Work out the finished part from the listing and answer in its coordinate system (mm). A direction names the side the tool comes from. Round coordinates to 2 decimals unless told otherwise and drop trailing zeros. Order: outer loops, then holes, each group sorted by start corner. A loop starts at its lowest first (then second) coordinate and runs counter-clockwise, first axis right, second up.
from build123d import *

# Parameters (mm, degrees)
F0_W     = 30
F0_H     = 30
F1_DEPTH = 2
F2_SIZE  = 0.5
F3_R     = 3.25
F4_DEPTH = 10
F5_SIZE  = 1


with BuildPart() as f1:
    # F0 (on Top) → F1 (new body)
    with BuildSketch(Plane.XY):
        Rectangle(F0_W, F0_H)
    extrude(amount=F1_DEPTH)

    # F2
    f2_edges = [f1.edges().sort_by_distance(p)[0] for p in [
        (-15, 0, 2),
        (0, 15, 2),
        (15, 0, 2),
        (0, -15, 2),
    ]]
    chamfer(f2_edges, length=F2_SIZE)

    # F3 (on Top) → F4 (join)
    with BuildSketch(Plane.XY):
        Circle(F3_R)
    extrude(amount=-F4_DEPTH)

    # F5
    f5_edges = [f1.edges().sort_by_distance(p)[0] for p in [
        (-3.25, 0, -10),
    ]]
    chamfer(f5_edges, length=F5_SIZE)


solid = f1.part
Item 1: Find section C-C (z = -4.5). Write down the section's boundary in (x, y), plus the area to 3 significant figures.
Item 2: A tool of negligible diameter and unlimited length cuts with its end or side. For faces 1 (the face through (0, 15, 1)), 2 (the face through (-2.579, -1.978, -4.437)), from which of +Z, -Z, +X, -X, +Y, -Y can it reach the whole face along a straight path? Write none if from no direction.
Item 3: Find section D-D (y = 9.75). Write down the section's boundary in (x, z).
Item 4: Given pin 1 (9 mm diameter, centred on x = -2, y = 5, fed in from -Z); pin 2 (4 mm diameter, centred on x = 3.5, z = -8.5, fed in from +Y), each flat-ended and moving along its own axis, determine where each tip first touches the part or whether it passes through.
Item 5: Find section A-A (y = 0). Write down the section's boundary in (x, z).
Item 6: Find the intervals of material crossed by line 1 along Z through (x, y) = (8, -10); line 2 along X through (y, z) = (1.75, -1.75); line 3 along X through (y, z) = (-0.25, -9), in increasing order.
Model answer:
1. outline: circle Ø6.5 at (0, 0)
1. area: 33.2 mm2
2. face 1: +Z, -Z, +X, -X, +Y
2. face 2: -Z
3. outline: (-15, 0) - (15, 0) - (15, 1.5) - (14.5, 2) - (-14.5, 2) - (-15, 1.5) - close
4. pin 1: stops at z = -10
4. pin 2: stops at y = 2.88
5. outline: (-15, 0) - (-3.25, 0) - (-3.25, -9) - (-2.25, -10) - (2.25, -10) - (3.25, -9) - (3.25, 0) - (15, 0) - (15, 1.5) - (14.5, 2) - (-14.5, 2) - (-15, 1.5) - close
6. line 1: z = 0 to 2
6. line 2: x = -2.74 to 2.74
6. line 3: x = -3.24 to 3.24
